For this review, take the finished solid that the model builds, in its own axes (mm). A direction names the side the tool comes from. Round coordinates to 2 decimals unless told otherwise and drop trailing zeros. Order: outer loops, then holes, each group sorted by start corner. A loop starts at its lowest first (then second) coordinate and runs counter-clockwise, first axis right, second up. Notation, with made-up numbers: (-8, -10) -> (22, -10) arc R4 ccw to (22, -6) -> close; hole circle Ø6 at (-28, 79.25). An arc over 180 degrees is marked (long way). Use a Markdown table: item, result. Add a question column.
1) Consider section B-B (y = 3). State the section outline as (x, z) points, plus the area to 3 significant figures.
2) Clearance check with flat-ended pins moving along their axes: P1, Ø1.3, axis at x = 1.5, y = -5, coming from the -Z side; P2, Ø2.5, axis at y = 0, z = 30.5, coming from the +X side; P3, Ø1, axis at x = -1.5, z = 22.5, coming from the +Y side. State where each tip first meets the part, or that it passes through.
3) Wall thickness on line 1 along Z through (x, y) = (3.75, -3.25); line 2 along Y through (x, z) = (4, 16.5); line 3 along Z through (x, y) = (4, 5): over which ranges is each line inside the solid? List them lowest first. Write a range as [from, to].
4) Draft analysis for pull direction X (two halves, no side actions). For faces 6 (the face through (-5, 0, 8)), 7 (the face through (-0.1, 6, 23.6)), 8 (the face through (4.595, -4.544, 19.649)), state which applies: pulls with the +X half, pulls with the -X half, needs draft (parallel to the pull), parting line crosses it, or undercut.
5) Consider section D-D (z = 7.5). State the section outline as (x, y) points, plus the area to 3 significant figures.
6) Consider section A-A (z = 17). State the section outline as (x, y) points.
7) Consider section C-C (x = 4). State the section outline as (y, z) points.
8) Machinability: for faces 1 (the face through (0, 2, 20)), 2 (the face through (0, 6, 7)), 3 (the face through (4, 5, 15.1)), 4 (the face through (-4, -5, 15.1)), 5 (the face through (1, 0, 28)), which of the approach directions +Z, -Z, +X, -X, +Y, -Y give a long, thin tool a straight path to every point of the face, cutting with its end or side? Answer none if there is none.
Autodesk Fusion 360 part; units mm, degrees
sketch "Sketch1" plane through (0, 0, 0) normal (0, 0, 1) x (1, 0, 0)
  circle A0 centre (0, 0) radius 6
  line L0 (-5, 6) -> (5, 6)
  line L1 (5, 6) -> (5, -6)
  line L2 (5, -6) -> (-5, -6)
  line L3 (-5, -6) -> (-5, 6)
  line L4 (-5, 6) -> (5, -6) construction
  line L5 (5, 6) -> (-5, -6) construction
  dimension "d1" = 12
  dimension "d2" = 10
  dimension "d3" = 12
extrude "Extrude1" add sketch "Sketch1" along normal blind 15.1 contours A0 L1 L3
sketch "Sketch2" plane through (0, 0, 15.1) normal (0, 0, 1) x (-1, 0, 0)
  arc A0 (-5, -3.3166) -> (5, -3.3166) centre (0, 0) ccw
  line L0 (5, -3.3166) -> (5, 3.3166)
  arc A1 (5, 3.3166) -> (-5, 3.3166) centre (0, 0) ccw
  line L1 (-5, 3.3166) -> (-5, -3.3166)
  line L2 (5, -6) -> (-5, -6)
  line L3 (-5, -6) -> (-5, 6)
  line L4 (-5, 6) -> (5, 6)
  line L5 (5, 6) -> (5, -6)
  line L6 (5, -6) -> (-5, 6) construction
  line L7 (-5, -6) -> (5, 6) construction
  dimension "d6" = 10
  dimension "d7" = 12
extrude "Extrude2" add sketch "Sketch2" along normal blind 9
sketch "Sketch3" plane through (0, 0, 24.1) normal (0, 0, 1) x (-1, 0, 0)
  line L0 (5, 6) -> (-5, 6)
  line L1 (-5, 6) -> (-5, -6)
  line L2 (-5, -6) -> (5, -6)
  line L3 (5, -6) -> (5, 6)
  circle A0 centre (0, 0) radius 2
  circle A1 centre (0, 0) radius 1.5
  dimension "d10" = 4
  dimension "d11" = 3
extrude "Extrude3" add sketch "Sketch3" along normal blind 0.8 contours A0
extrude "Extrude4" add 1 faces at (-0.567, 0.5383, 24.1) along direction (0, 0, 1) blind 10
extrude "Extrude5" add sketch "Sketch3" along normal blind 10 contours A1
sketch "Sketch4" plane through (0, 0, 0) normal (0, 0, -1) x (1, 0, 0)
  arc A0 (-5, -3.3166) -> (5, -3.3166) centre (0, 0) ccw
  line L0 (5, -3.3166) -> (5, 3.3166)
  arc A1 (5, 3.3166) -> (-5, 3.3166) centre (0, 0) ccw
  line L1 (-5, 3.3166) -> (-5, -3.3166)
  circle A2 centre (0, 0) radius 2.5
  dimension "d18" = 5
extrude "Extrude6" add sketch "Sketch4" along normal blind 1.2 contours A2
sketch "Sketch5" plane through (0, 0, 24.1) normal (0, 0, 1) x (-1, 0, 0)
  line L0 (-4, 5) -> (4, 5)
  line L1 (4, 5) -> (4, -5)
  line L2 (4, -5) -> (-4, -5)
  line L3 (-4, -5) -> (-4, 5)
  line L4 (-4, 5) -> (4, -5) construction
  line L5 (4, 5) -> (-4, -5) construction
  circle A0 centre (4, -5) radius 0.75
  circle A1 centre (-4, -5) radius 0.75
  circle A2 centre (4, 5) radius 0.75
  circle A3 centre (-4, 5) radius 0.75
  circle A4 centre (0, 0) radius 1.5
  dimension "d21" = 1.5
  dimension "d22" = 1.5
  dimension "d23" = 1.5
  dimension "d24" = 1.5
  dimension "d25" = 3
extrude "Extrude7" cut 1 faces at (0.0498, 4.6648, 24.1) along direction (0, 0, -1) blind 7 from surface at 1
extrude "Extrude8" add sketch "Sketch5" against normal blind 8.5 contours L0 L3 A3 | L0 L3 A3 | L0 L1 A2 | L0 L1 A2 | L2 L3 A1 | L2 L3 A1 | L1 L2 A0 | L1 L2 A0 | A4
sketch "Sketch6" plane through (0, 0, 0) normal (0, 1, 0) x (1, 0, 0)
  line L0 (1, -28) -> (3, -28)
  line L1 (3, -28) -> (3, -35)
  line L2 (3, -35) -> (1, -35)
  line L3 (1, -35) -> (1, -28)
sketch "Sketch7" plane through (0, 0, 0) normal (0, 1, 0) x (1, 0, 0)
extrude "Extrude9" cut sketch "Sketch6" along normal blind 8
sketch "Sketch8" plane through (0, 0, 0) normal (0, 1, 0) x (1, 0, 0)
  line L0 (0.4932, -34.2266) -> (2, -34.2266)
  line L1 (2, -34.2266) -> (2, -28)
  line L2 (2, -28) -> (0.4932, -28)
  line L3 (0.4932, -28) -> (0.4932, -34.2266)
extrude "Extrude10" cut sketch "Sketch8" along normal blind 100
extrude "Extrude11" cut sketch "Sketch8" against normal blind 100
Results list:
| question | item | result |
|---|---|---|
| 1 | outline | (-5, 0) -> (5, 0) -> (5, 16.1) -> (-5, 16.1) -> close; (-5, 23.1) -> (5, 23.1) -> (5, 24.1) -> (-5, 24.1) -> close |
| 1 | area | 171 mm2 |
| 2 | P1 | z = 0 |
| 2 | P2 | x = 0.49 |
| 2 | P3 | y = 1.73 |
| 3 | line 1 | [0, 16.1], [23.1, 24.1] |
| 3 | line 2 | [-5.75, -4.25], [4.25, 5.75] |
| 3 | line 3 | [15.1, 24.1] |
| 4 | face 6 | pulls with the -X half |
| 4 | face 7 | needs draft |
| 4 | face 8 | undercut |
| 5 | outline | (-5, -3.32) arc R6 ccw to (5, -3.32) -> (5, 3.32) arc R6 ccw to (-5, 3.32) -> close |
| 5 | area | 104 mm2 |
| 6 | outline | circle Ø1.5 at (-4, -5); circle Ø1.5 at (-4, 5); circle Ø4 at (0, 0); circle Ø1.5 at (4, -5); circle Ø1.5 at (4, 5) |
| 7 | outline | (-6, 15.1) -> (-4.47, 15.1) -> (-4.47, 0) -> (4.47, 0) -> (4.47, 15.1) -> (6, 15.1) -> (6, 16.1) -> (5.75, 16.1) -> (5.75, 23.1) -> (6, 23.1) -> (6, 24.1) -> (-6, 24.1) -> (-6, 23.1) -> (-5.75, 23.1) -> (-5.75, 16.1) -> (-6, 16.1) -> close; hole (-4.25, 16.1) -> (4.25, 16.1) -> (4.25, 23.1) -> (-4.25, 23.1) -> close |
| 8 | face 1 | none |
| 8 | face 2 | -Z, +Y |
| 8 | face 3 | -Z, +X, +Y |
| 8 | face 4 | -Z, -X, -Y |
| 8 | face 5 | +Z, +X, +Y, -Y |
